```python
from build123d import *

# Parameters (mm, degrees)
SKETCH1_W           = 57
SKETCH1_H           = 57
BOSS_EXTRUDE1_DEPTH = 18
FILLET1_R           = 5
FILLET2_R           = 10


with BuildPart() as part:
    # Sketch1 → Boss-Extrude1 (new body)
    with BuildSketch(Plane(origin=(0, 0, 0), x_dir=(1, 0, 0), z_dir=(0, 1, 0))):
        with Locations((28.5, 28.5)):
            Rectangle(SKETCH1_W, SKETCH1_H)
    extrude(amount=BOSS_EXTRUDE1_DEPTH)

    # Fillet1
    fillet1_edges = [part.edges().sort_by_distance(p)[0] for p in [
        (57, 9, 0),
    ]]
    fillet(fillet1_edges, radius=FILLET1_R)

    # Fillet2
    fillet2_edges = [part.edges().sort_by_distance(p)[0] for p in [
        (0, 9, -57),
        (57, 9, -57),
        (0, 9, 0),
    ]]
    fillet(fillet2_edges, radius=FILLET2_R)


solid = part.part
```
Work out the finished part from the listing and answer in its coordinate system (mm). Coordinates: 2 decimals unless noted, no trailing zeros. Loops run counter-clockwise (first coordinate to the right, second up) from the corner with the lowest first, then second, coordinate; pieces in that order, holes last. Notation, with made-up numbers: (-34, 82.25) - (12, 82.25) arc R20 cw to (12, 118.25) - close; hole circle Ø10 at (54.25, 76). An arc over 180 degrees is marked (long way). Use a Markdown table: item, result.
Item 1: Consider probe 1 along X at (y, z) = (12.25, -49); probe 2 along X at (y, z) = (8.75, -47.5); probe 3 along Z at (x, y) = (52, 6.75). Determine where each line is inside the solid, lowest interval first. Write a range as from..to.
Evaluation:
| item | result |
|---|---|
| probe 1 | x = 0.2..56.8 |
| probe 2 | x = 0.01..56.99 |
| probe 3 | z = -55.66..0 |
Item 2: Find section B-B, the plane x = 4. Determine the outline of the cut face in (y, z).
Evaluation:
| item | result |
|---|---|
| outline | (0, -55) - (18, -55) - (18, -2) - (0, -2) - close |
Item 3: Find section C-C, the plane z = -51.5. Determine the outline of the cut face in (x, y), and give its area (3 significant figures).
Evaluation:
| item | result |
|---|---|
| outline | (1.07, 0) - (55.93, 0) - (55.93, 18) - (1.07, 18) - close |
| area | 987 mm2 |
Item 4: Given pin 1 Ø6 at (x, z) = (41.5, -25.5) entering from -Y, flat-ended and moving along its own axis, determine where the tip first touches the part or whether it passes through.
Evaluation:
| item | result |
|---|---|
| pin 1 | stops at y = 0 |
Item 5: Find section A-A, the plane y = 12. Determine the outline of the cut face in (x, z).
Evaluation:
| item | result |
|---|---|
| outline | (0, -47) arc R10 ccw to (10, -57) - (47, -57) arc R10 ccw to (57, -47) - (57, -5) arc R5 ccw to (52, 0) - (10, 0) arc R10 ccw to (0, -10) - close |
